from build123d import *

# Parameters (mm, degrees)
EXTRUDE_2_DEPTH          = 110
SHELL_5_T                = 5
SKETCH_2_W               = 69.117640956
SKETCH_2_H               = 110
CUT_EXTRUDE_2_DEPTH      = 5
CUT_EXTRUDE_5_DEPTH      = 188.422981916
CUT_EXTRUDE_5_DEPTH_BACK = 188.422981916
SKETCH_3_R               = 1.5
FILLET_2_R               = 5


with BuildPart() as part:
    # 草图1 → 凸台-拉伸2 (new body)
    with BuildSketch(Plane.XY):
        with BuildLine():
            Line((0, 0), (0, 71.515747703))
            Line((0, 71.515747703), (64.301044277, 93.881328321))
            Line((64.301044277, 93.881328321), (103.260442774, -18.126942356))
            ThreePointArc((103.260442774, -18.126942356), (49.31823123, -22.233763367), (0, 0))
        make_face()
    extrude(amount=EXTRUDE_2_DEPTH)

    # 抽壳5
    shell_5_openings = [part.faces().sort_by_distance(p)[0] for p in [
        (83.780743525, 37.877192982, 55),
    ]]
    offset(amount=SHELL_5_T, openings=shell_5_openings, kind=Kind.INTERSECTION)

    # 草图2 → 切除-拉伸2 (cut)
    with BuildSketch(Plane(origin=(-23.832986898, 68.51983733, 0), x_dir=(0.9444967967061592, 0.32852062494127277, 0), z_dir=(-0.3285206249412727, 0.944496796706159, 0))):
        with Locations((57.015262517, -55)):
            Rectangle(SKETCH_2_W, SKETCH_2_H)
    extrude(amount=-CUT_EXTRUDE_2_DEPTH, mode=Mode.SUBTRACT)

    # 草图3 → 切除-拉伸5 (cut, two sides: drawn at the far end of the back side and taken through both)
    with BuildSketch(Plane.XY.offset(115).offset(-CUT_EXTRUDE_5_DEPTH_BACK)):
        with Locations((11, 73.245743445)):
            Circle(SKETCH_3_R)
        with Locations((6, 61.732695858)):
            Circle(SKETCH_3_R)
    extrude(amount=CUT_EXTRUDE_5_DEPTH + CUT_EXTRUDE_5_DEPTH_BACK, mode=Mode.SUBTRACT)

    # 圆角2
    fillet_2_edges = [part.edges().sort_by_distance(p)[0] for p in [
        (103.260442774, -18.126942356, 55),
    ]]
    fillet(fillet_2_edges, radius=FILLET_2_R)


solid = part.part
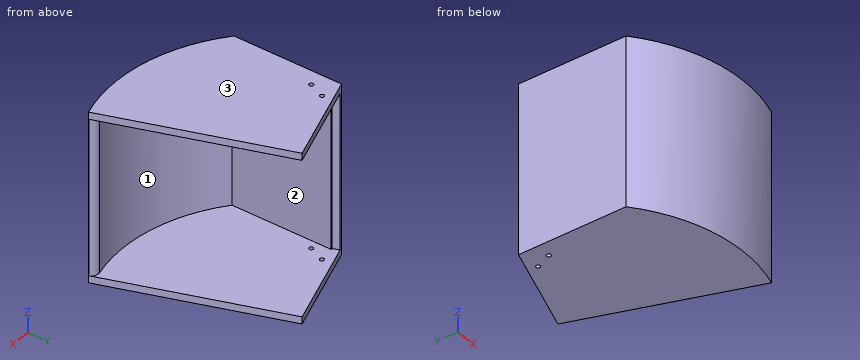
Work out the finished part from the listing and answer in its coordinate system (mm). Face numbers are marked on the shaded views. Round coordinates to 2 decimals unless told otherwise and drop trailing zeros. Loops run counter-clockwise (first coordinate to the right, second up) from the corner with the lowest first, then second, coordinate; pieces in that order, holes last. Notation, with made-up numbers: M -29,23 L -21,23 A21 cw -21,54 Z; hole C 56.25,57.5 d4. An arc over 180 degrees is marked long. One line per question, with ' | ' between items. Start each with the question number.
(1) A cutting plane is placed at B-B on x = 47.5. Write down the section's boundary in (y, z), plus the area to 3 significant figures.
(2) Find the intervals of material crossed by line 1 (Z direction, x = 65.5, y = 46); line 2 (X direction, y = 16, z = 47.5); line 3 (Y direction, x = 68.5, z = 71), in increasing order.
(3) For a pull along X with two mould halves and no side action, classify the marked faces 1, 2 and 3 as released by +X, released by -X, zero draft, split by the parting line, or undercut.
(4) Flat-ended cylindrical pins translate along their axes: pin 1 Ø2.5 at (x, y) = (6, 61.73) entering from -Z; pin 2 Ø5 at (x, y) = (11, 73.25) entering from +Z; pin 3 Ø1 at (x, z) = (14.5, 27) entering from -Y; pin 4 Ø10 at (x, z) = (61.5, 30) entering from +Y. Find the tip coordinate at first contact, or state that the pin passes through.
(5) A cutting plane is placed at C-C on z = 54.5. Write down the section's boundary in (x, y), plus the area to 3 significant figures.
(6) A cutting plane is placed at A-A on y = 46. Write down the section's boundary in (x, z), plus the area to 3 significant figures.
Geometry check:
1) outline: M -26.99,-5 L 93.33,-5 L 93.33,0 L -21.9,0 L -21.9,110 L 93.33,110 L 93.33,115 L -26.99,115 Z | area: 1,760 mm²
2) line 1: z = -5 to 0, 110 to 115 | line 2: x = -5 to 0 | line 3: y = -28.88 to -23.88
3) face 1: undercut | face 2: released by +X | face 3: zero draft
4) pin 1: passes through | pin 2: stops at z = 115 | pin 3: stops at y = -15.74 | pin 4: stops at y = -23.25
5) outline: M -5,-2.37 A114.43 ccw 104.9,-22.85 L 104.85,-22.71 A5 ccw 98.74,-19.55 A109.43 cw 0,0 L 0,71.52 L -0.98,71.17 L -2.62,75.9 L -5,75.07 Z | area: 937 mm²
6) outline: M -5,-5 L 80.96,-5 L 80.96,0 L 0,0 L 0,110 L 80.96,110 L 80.96,115 L -5,115 Z | area: 1,410 mm²
